Read the model definition and answer for the solid it produces. Units are mm, in the model's axes. Give positions to 0.01 mm unless a question says otherwise; leave off trailing zeros. Order: outer loops, then holes, each group sorted by start corner. A loop starts at its lowest first (then second) coordinate and runs counter-clockwise, first axis right, second up. Notation, with made-up numbers: (-6, 35) - (45, 35) arc R13 cw to (45, 54) - close; hole circle Ø3 at (-38.5, -31.5). An arc over 180 degrees is marked (long way). Use a Markdown table: item, result. Add a question column.
1. A cutting plane is placed at C-C on y = 0. Determine the outline of the cut face in (x, z), and give its area (3 significant figures).
2. A cutting plane is placed at B-B on z = 9.25. Determine the outline of the cut face in (x, y).
3. A flat-ended cylindrical pin translates along its axis: P1, Ø9, axis at x = 202, y = 0, coming from the -Z side. Find the tip coordinate at first contact, or state that the pin passes through.
4. Consider L1, parallel to Y at x = -202, z = -6.75; L2, parallel to X at y = 2.25, z = 5.25; L3, parallel to X at y = -2.75, z = -11.5. Determine where each line is inside the solid, lowest interval first.
5. A cutting plane is placed at A-A on x = 0. Determine the outline of the cut face in (y, z), and give its area (3 significant figures).
```python
from build123d import *

# Parameters (mm, degrees)
SKETCH1_W           = 434
SKETCH1_H           = 30
SKETCH1_R           = 7.5
BOSS_EXTRUDE1_DEPTH = 15


with BuildPart() as part:
    # Sketch1 → Boss-Extrude1 (new, symmetric)
    with BuildSketch(Plane.XY):
        Rectangle(SKETCH1_W, SKETCH1_H)
        with Locations((-202, 0)):
            Circle(SKETCH1_R, mode=Mode.SUBTRACT)
        with Locations((202, 0)):
            Circle(SKETCH1_R, mode=Mode.SUBTRACT)
        Circle(SKETCH1_R, mode=Mode.SUBTRACT)
    extrude(amount=BOSS_EXTRUDE1_DEPTH, both=True)


solid = part.part
```
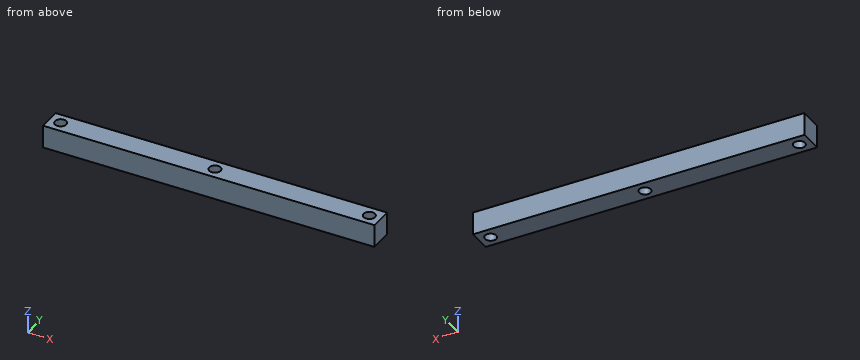
Output values:
| question | item | result |
|---|---|---|
| 1 | outline | (-217, -15) - (-209.5, -15) - (-209.5, 15) - (-217, 15) - close; (-194.5, -15) - (-7.5, -15) - (-7.5, 15) - (-194.5, 15) - close; (7.5, -15) - (194.5, -15) - (194.5, 15) - (7.5, 15) - close; (209.5, -15) - (217, -15) - (217, 15) - (209.5, 15) - close |
| 1 | area | 11,700 mm² |
| 2 | outline | (-217, -15) - (217, -15) - (217, 15) - (-217, 15) - close; hole circle Ø15 at (-202, 0); hole circle Ø15 at (0, 0); hole circle Ø15 at (202, 0) |
| 3 | P1 | through |
| 4 | L1 | -15 to -7.5, 7.5 to 15 |
| 4 | L2 | -217 to -209.15, -194.85 to -7.15, 7.15 to 194.85, 209.15 to 217 |
| 4 | L3 | -217 to -208.98, -195.02 to -6.98, 6.98 to 195.02, 208.98 to 217 |
| 5 | outline | (-15, -15) - (-7.5, -15) - (-7.5, 15) - (-15, 15) - close; (7.5, -15) - (15, -15) - (15, 15) - (7.5, 15) - close |
| 5 | area | 450 mm² |
